from build123d import *

# Parameters (mm, degrees)
F0_R     = 25
F1_DEPTH = 560
F2_R     = 12.5
F3_DEPTH = 25.5
F4_R     = 12.5
F5_DEPTH = 25.5


with BuildPart() as f1:
    # F0 (on Right) → F1 (new body)
    with BuildSketch(Plane.YZ):
        Circle(F0_R)
    extrude(amount=F1_DEPTH)

    # F2 (on face) → F3 (cut)
    with BuildSketch(Plane(origin=(0, 0, 0), x_dir=(0, -1, 0), z_dir=(-1, 0, 0))):
        Circle(F2_R)
    extrude(amount=-F3_DEPTH, mode=Mode.SUBTRACT)

    # F4 (on face) → F5 (cut)
    with BuildSketch(Plane.YZ.offset(560)):
        Circle(F4_R)
    extrude(amount=-F5_DEPTH, mode=Mode.SUBTRACT)


solid = f1.part
Source: CAD feature listing. Evaluate the final solid. Frame: model axes, mm. A direction names the side the tool comes from. Give positions to 0.01 mm unless a question says otherwise; leave off trailing zeros. Write each loop counter-clockwise with the first axis right and the second up, starting at its lowest first coordinate (ties: lowest second). Pieces come first, ordered by that corner, then holes. Notation, with made-up numbers: (3, 55) -> (57, 55) arc R19 cw to (57, 59) -> close; hole circle Ø7 at (6, -2). An arc over 180 degrees is marked (long way). Return JSON: item names as keys, results as strings. Group by question number.
1. Pin query (flat end, axial travel): pin 1 Ø4 at (y, z) = (-3, 1) entering from -X; pin 2 Ø1 at (x, z) = (228.5, -6) entering from +Y; pin 3 Ø6 at (x, y) = (174, -15) entering from +Z. Return the tip coordinate at first contact, or that it passes through.
2. Access query for faces 4 (the face through (534.5, 0, 0)), 5 (the face through (12.572, -11.923, 3.755)), 6 (the face through (560, -11.5, 5.9)). Directions: +Z, -Z, +X, -X, +Y, -Y. A direction counts if a zero-diameter tool reaches every point of the face in a straight line with its end or side. Return the directions, or none.
3. Material intervals for line 1 (Z direction, x = 8.5, y = 0); line 2 (X direction, y = 2, z = 5); line 3 (Z direction, x = 424, y = -16), sorted ascending. Write a range as from..to.
4. Mould query, pull axis Y, two halves, no side actions, for faces 1 (the face through (25.5, 0, 0)), 2 (the face through (276.08, 23.846, 7.509)), 3 (the face through (0, -11.5, 5.9)). Classes: +Y half, -Y half, draft (parallel to the pull), parting line (faces both ways), or undercut.
5. Section C-C, the plane x = 49. Output: boundary loops of the cut face in (y, z), then the cut area to 3 significant figures.
6. Section A-A, the plane z = 0. Output: boundary loops of the cut face in (x, y), then the cut area to 3 significant figures.
Determined:
{
 "1": {"pin 1": "stops at x = 25.5", "pin 2": "stops at y = 24.39", "pin 3": "stops at z = 21.93"},
 "2": {"face 4": "+X", "face 5": "-X", "face 6": "+Z, -Z, +X, +Y, -Y"},
 "3": {"line 1": "z = -25..-12.5, 12.5..25", "line 2": "x = 25.5..534.5", "line 3": "z = -19.21..19.21"},
 "4": {"face 1": "undercut", "face 2": "parting line", "face 3": "draft"},
 "5": {"outline": "circle Ø50 at (0, 0)", "area": "1,960 mm2"},
 "6": {"outline": "(0, -25) -> (560, -25) -> (560, -12.5) -> (534.5, -12.5) -> (534.5, 12.5) -> (560, 12.5) -> (560, 25) -> (0, 25) -> (0, 12.5) -> (25.5, 12.5) -> (25.5, -12.5) -> (0, -12.5) -> close", "area": "26,700 mm2"}
}
